The model under review builds one solid part; all positions refer to its coordinate system, in mm. A direction names the side the tool comes from. Coordinates: 2 decimals unless noted, no trailing zeros. Order: outer loops, then holes, each group sorted by start corner. A loop starts at its lowest first (then second) coordinate and runs counter-clockwise, first axis right, second up.
```python
from build123d import *

# Parameters (mm, degrees)
SZKIC1_W                    = 4
SZKIC1_H                    = 1
DODANIE_WYCI_GNI_CIE1_DEPTH = 10
SZKIC2_R                    = 0.5
WYTNIJ_WYCI_GNI_CIE1_DEPTH  = 10
SZKIC3_W                    = 4
SZKIC3_H                    = 1
DODANIE_WYCI_GNI_CIE2_DEPTH = 1
SZKIC4_W                    = 3.2
SZKIC4_H                    = 0.5
DODANIE_WYCI_GNI_CIE3_DEPTH = 3.9
SZKIC5_R                    = 1
WYTNIJ_WYCI_GNI_CIE2_DEPTH  = 3.9
ZAOKR_GLENIE1_R             = 0.25


with BuildPart() as part:
    # Szkic1 → Dodanie-wyciągnięcie1 (new body)
    with BuildSketch(Plane(origin=(0, 0, 0), x_dir=(1, 0, 0), z_dir=(0, 1, 0))):
        Rectangle(SZKIC1_W, SZKIC1_H)
    extrude(amount=DODANIE_WYCI_GNI_CIE1_DEPTH)

    # Szkic2 → Wytnij-wyciągnięcie1 (cut)
    with BuildSketch(Plane(origin=(0, 0, -0.5), x_dir=(-1, 0, 0), z_dir=(0, 0, -1))):
        with Locations((0, 7)):
            Circle(SZKIC2_R)
    extrude(amount=-WYTNIJ_WYCI_GNI_CIE1_DEPTH, mode=Mode.SUBTRACT)

    # Szkic3 → Dodanie-wyciągnięcie2 (add)
    with BuildSketch(Plane.XY.offset(0.5)):
        with Locations((0, 9.5)):
            Rectangle(SZKIC3_W, SZKIC3_H)
    extrude(amount=DODANIE_WYCI_GNI_CIE2_DEPTH)

    # Szkic4 → Dodanie-wyciągnięcie3 (add)
    with BuildSketch(Plane(origin=(0, 0, 0), x_dir=(-1, 0, 0), z_dir=(0, -1, 0))):
        Rectangle(SZKIC4_W, SZKIC4_H)
    extrude(amount=DODANIE_WYCI_GNI_CIE3_DEPTH)

    # Szkic5 → Wytnij-wyciągnięcie2 (cut)
    with BuildSketch(Plane.XY.offset(0.25)):
        with Locations((0, -2.4)):
            Circle(SZKIC5_R)
    extrude(amount=-WYTNIJ_WYCI_GNI_CIE2_DEPTH, mode=Mode.SUBTRACT)

    # Zaokrąglenie1
    zaokr_glenie1_edges = [part.edges().sort_by_distance(p)[0] for p in [
        (-1.6, 0, 0),
        (0, 0, -0.25),
        (1.6, 0, 0),
        (0, 0, 0.25),
        (-1.6, -3.9, 0),
        (1.6, -3.9, 0),
    ]]
    fillet(zaokr_glenie1_edges, radius=ZAOKR_GLENIE1_R - 0.0001)  # a hair under: the kernel refuses the full size


solid = part.part
```
(1) We need section B-B, the plane x = 0. Count the separate pieces of the cut face and the enclosed holes in it, and give its area (3 significant figures).
A:
separate pieces: 3
enclosed holes: 0
area: 11.0 mm2
(2) For pin 1 Ø2 at (x, y) = (0.5, 6.5) entering from +Z; pin 2 Ø0.5 at (x, z) = (-1, 1) entering from -Y; pin 3 Ø0.6 at (y, z) = (-2.5, 0) entering from -X, all flat-tipped, find the tip position at first contact; note any pin that passes through.
A:
pin 1: stops at z = 0.5
pin 2: stops at y = 9
pin 3: stops at x = -1.6
(3) Wall thickness on probe 1 along Y at (x, z) = (0, -0.05); probe 2 along Z at (x, y) = (0.5, 3.5); probe 3 along Y at (x, z) = (1.05, 1.4): over which ranges is each line inside the solid? List them lowest first.
A:
probe 1: y = -3.9 to -3.4, -1.4 to 6.5, 7.5 to 10
probe 2: z = -0.5 to 0.5
probe 3: y = 9 to 10
(4) Draft analysis for pull direction X (two halves, no side actions). For faces 1 (the face through (0.108, 6.512, -0.007)), 2 (the face through (2, 5, 0)), 3 (the face through (0, 10, 0)), state which applies: released by +X, released by -X, zero draft, split by the parting line, or undercut.
A:
face 1: undercut
face 2: released by +X
face 3: zero draft
(5) Machinability: for faces 4 (the face through (0, 5, -0.5)), 5 (the face through (0, -1, 0.25)), 6 (the face through (0, -1, -0.25)), which of the approach directions +Z, -Z, +X, -X, +Y, -Y give a long, thin tool a straight path to every point of the face, cutting with its end or side? Answer none if there is none.
A:
face 4: -Z, +X, -X, +Y, -Y
face 5: +Z, +X, -X, -Y
face 6: -Z, +X, -X, -Y
(6) We need section A-A, the plane y = 7. Write out the cut boundary in (x, z), and give its area (3 significant figures).
A:
outline: (-2, -0.5) - (-0.5, -0.5) - (-0.5, 0.5) - (-2, 0.5) - close; (0.5, -0.5) - (2, -0.5) - (2, 0.5) - (0.5, 0.5) - close
area: 3.00 mm2
(7) We need section D-D, the plane y = -2.4. Write out the cut boundary in (x, z).
A:
outline: (-1.6, -0.25) - (-1, -0.25) - (-1, 0.25) - (-1.6, 0.25) - close; (1, -0.25) - (1.6, -0.25) - (1.6, 0.25) - (1, 0.25) - close
